Verification items for this drawing (mm, ordinates from the low corner). A direction names the side the tool comes from. Coordinates: 2 decimals unless noted, no trailing zeros. Order: outer loops, then holes, each group sorted by start corner. A loop starts at its lowest first (then second) coordinate and runs counter-clockwise, first axis right, second up. Notation, with made-up numbers: (10, -33.75) - (23, -33.75) arc R31 ccw to (23, -8.75) - close; hole circle Ø7 at (-16.75, 13.25). An arc over 180 degrees is marked (long way). One line per question, with ' | ' between items. Start each with the question number.
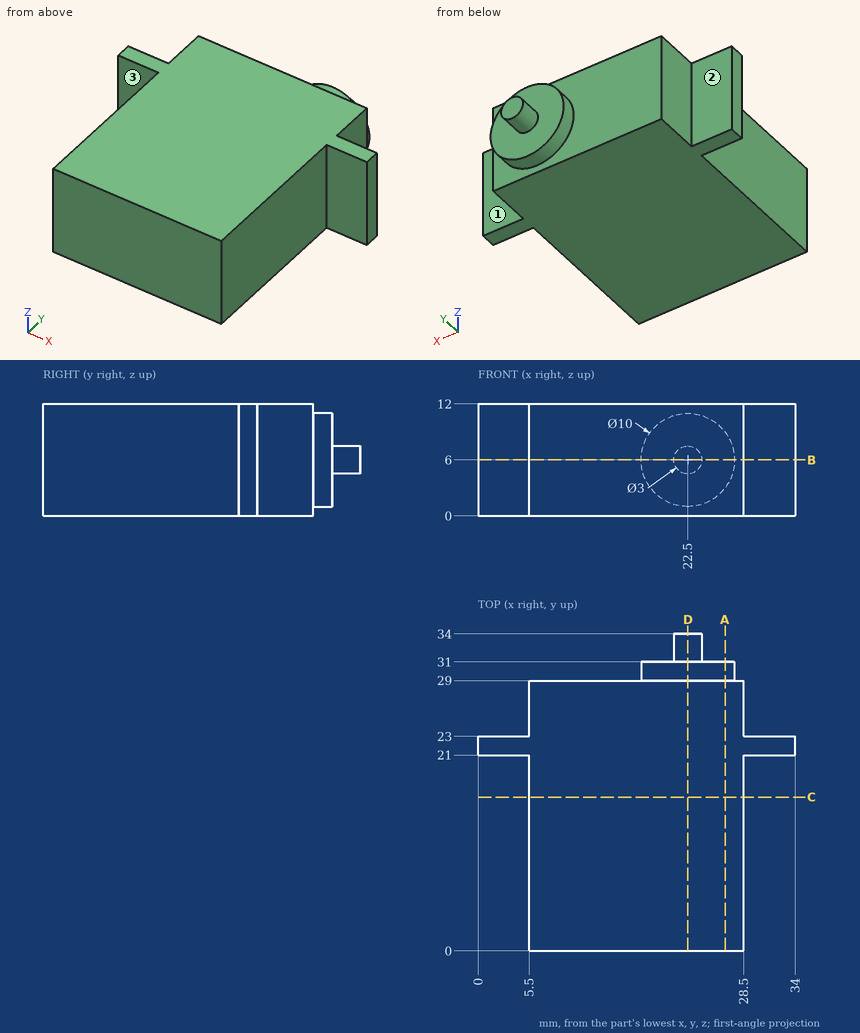
Item 1: Section check C-C (y = 16.5). Record the cut outline in (x, z), then the cut area to 3 significant figures.
Item 2: Set-up check for the marked faces 1, 2 and 3: record each of +Z, -Z, +X, -X, +Y, -Y from which the full face is reachable in a straight line by a thin tool's end or side.
Item 3: Section check B-B (z = 6). Record the cut outline in (x, y), then the cut area to 3 significant figures.
Item 4: Section check A-A (x = 26.5). Record the cut outline in (y, z).
Item 5: Section check D-D (x = 22.5). Record the cut outline in (y, z).
Item 6: Thickness scan on probe 1 along Y at (x, z) = (13, 4.75); probe 2 along Y at (x, z) = (18, 5.25); probe 3 along X at (y, z) = (14.5, 10). Record the ranges inside material, lowest first. Write a range as from..to.
Item 7: Gauge pin test, flat ends, axial feed: pin 1 (3 mm diameter, centred on x = 1.5, z = 5, fed in from -Y); pin 2 (6 mm diameter, centred on x = 32.5, z = 7.5, fed in from +Y); pin 3 (1 mm diameter, centred on y = 12, z = 4.5, fed in from -X); pin 4 (6 mm diameter, centred on x = 30, z = 3, fed in from -Y). Record the tip position at first contact, or that the pin passes through.
Completed:
1) outline: (5.5, 0) - (28.5, 0) - (28.5, 12) - (5.5, 12) - close | area: 276 mm^2
2) face 1: +Z, -Z, +X, +Y | face 2: +Z, -Z, -X, +Y | face 3: +Z, -Z, -X, -Y
3) outline: (0, 21) - (5.5, 21) - (5.5, 0) - (28.5, 0) - (28.5, 21) - (34, 21) - (34, 23) - (28.5, 23) - (28.5, 29) - (27.5, 29) - (27.5, 31) - (24, 31) - (24, 34) - (21, 34) - (21, 31) - (17.5, 31) - (17.5, 29) - (5.5, 29) - (5.5, 23) - (0, 23) - close | area: 718 mm^2
4) outline: (0, 0) - (29, 0) - (29, 3) - (31, 3) - (31, 9) - (29, 9) - (29, 12) - (0, 12) - close
5) outline: (0, 0) - (29, 0) - (29, 1) - (31, 1) - (31, 4.5) - (34, 4.5) - (34, 7.5) - (31, 7.5) - (31, 11) - (29, 11) - (29, 12) - (0, 12) - close
6) probe 1: y = 0..29 | probe 2: y = 0..31 | probe 3: x = 5.5..28.5
7) pin 1: stops at y = 21 | pin 2: stops at y = 23 | pin 3: stops at x = 5.5 | pin 4: stops at y = 0
